Check sheet for the modelled part. Datum: model origin and axes. Units: mm. A direction names the side the tool comes from. Coordinates: 2 decimals unless noted, no trailing zeros. Loops run counter-clockwise (first coordinate to the right, second up) from the corner with the lowest first, then second, coordinate; pieces in that order, holes last. Notation, with made-up numbers: (-34, 89) - (-11, 89) arc R17 ccw to (-11, 112) - close; hole circle Ø2 at (35, -7). An arc over 180 degrees is marked (long way). Answer as a JSON object with one key per item and string values. Group by question number.
from build123d import *

# Parameters (mm, degrees)
F0_W     = 32
F0_H     = 16
F1_DEPTH = 8
F2_R     = 2.5
F3_DEPTH = 2
F4_T     = -1.5


with BuildPart() as f1:
    # F0 (on Top) → F1 (new body)
    with BuildSketch(Plane.XY):
        Rectangle(F0_W, F0_H)
    extrude(amount=F1_DEPTH)

    # F2 (on face) → F3 (join)
    with BuildSketch(Plane.XY.offset(8)):
        with Locations((-12, 4)):
            Circle(F2_R)
        with Locations((-3.9529362693, 3.9800377563)):
            Circle(F2_R)
        with Locations((3.9575416595, 3.9243297651)):
            Circle(F2_R)
        with Locations((11.8680195883, 3.8129147142)):
            Circle(F2_R)
        with Locations((-11.9748292491, -3.8190248888)):
            Circle(F2_R)
        with Locations((-3.9529362693, -3.8747326471)):
            Circle(F2_R)
        with Locations((3.9575416595, -3.9861481637)):
            Circle(F2_R)
        with Locations((11.9237266481, -3.9861481637)):
            Circle(F2_R)
    extrude(amount=F3_DEPTH)

    # F4
    f4_openings = [f1.faces().sort_by_distance(p)[0] for p in [
        (0, 0, 0),
    ]]
    offset(amount=F4_T, openings=f4_openings, kind=Kind.INTERSECTION)


solid = f1.part
1. Material ranges on line 1 (Y direction, x = -12, z = 7.15); line 2 (X direction, y = 0.25, z = 4.5); line 3 (X direction, y = -4.25, z = 9.5), recorded low to high.
2. Sectioned sample at A-A on z = 5. Record the cut outline in (x, y), plus the area to 3 significant figures.
3. Sectioned sample at D-D on x = -12. Record the cut outline in (y, z).
4. Release check for a two-part mould opening along Y. For faces 1 (the face through (0, -8, 4)), 2 (the face through (3.22, 4.6, 7.49)), 3 (the face through (4, 4, 10)) record: released by +Y, released by -Y, zero draft, split by the parting line, or undercut.
5. Sectioned sample at C-C on x = 7. Record the cut outline in (y, z).
6. Sectioned sample at B-B on y = 1. Record the cut outline in (x, z), plus the area to 3 significant figures.
7. Gauge pin test, flat ends, axial feed: pin 1 (1.6 mm diameter, centred on x = 4.5, y = 4.5, fed in from -Z); pin 2 (0.6 mm diameter, centred on x = -12.5, y = -4, fed in from -Z); pin 3 (4 mm diameter, centred on x = -7.5, y = 1, fed in from +Z). Record the tip position at first contact, or that the pin passes through.
8. Access from +Z, -Z, +X, -X, +Y, -Y to the whole of each face (thin tool, end or side, straight path). Record for faces 4 (the face through (12.406, 4.656, 7.486)), 5 (the face through (1.974, -5.507, 8.986)), 6 (the face through (-16, 0, 4)).
Answers follow:
{
 "1": {"line 1": "y = -8 to -4.82, -2.82 to 3, 5 to 8", "line 2": "x = -16 to -14.5, 14.5 to 16", "line 3": "x = -14.44 to -9.51, -6.42 to -1.48, 1.47 to 6.44, 9.44 to 14.41"},
 "2": {"outline": "(-16, -8) - (16, -8) - (16, 8) - (-16, 8) - close; hole (-14.5, -6.5) - (14.5, -6.5) - (14.5, 6.5) - (-14.5, 6.5) - close", "area": "135 mm^2"},
 "3": {"outline": "(-8, 0) - (-6.5, 0) - (-6.5, 6.5) - (-4.82, 6.5) - (-4.82, 8.5) - (-2.82, 8.5) - (-2.82, 6.5) - (3, 6.5) - (3, 8.5) - (5, 8.5) - (5, 6.5) - (6.5, 6.5) - (6.5, 0) - (8, 0) - (8, 8) - (6.5, 8) - (6.5, 10) - (1.5, 10) - (1.5, 8) - (-1.32, 8) - (-1.32, 10) - (-6.32, 10) - (-6.32, 8) - (-8, 8) - close"},
 "4": {"face 1": "released by -Y", "face 2": "undercut", "face 3": "zero draft"},
 "5": {"outline": "(-8, 0) - (-6.5, 0) - (-6.5, 6.5) - (6.5, 6.5) - (6.5, 0) - (8, 0) - (8, 8) - (-8, 8) - close"},
 "6": {"outline": "(-16, 0) - (-14.5, 0) - (-14.5, 6.5) - (14.5, 6.5) - (14.5, 0) - (16, 0) - (16, 8) - (-16, 8) - close", "area": "67.5 mm^2"},
 "7": {"pin 1": "stops at z = 6.5", "pin 2": "stops at z = 8.5", "pin 3": "stops at z = 8"},
 "8": {"face 4": "-Z", "face 5": "+Z", "face 6": "+Z, -Z, -X, +Y, -Y"}
}
